Could you check a few things on this model? Use its own coordinates, in mm. A direction names the side the tool comes from. Coordinates: 2 decimals unless noted, no trailing zeros. Order: outer loops, then holes, each group sorted by start corner. A loop starts at its lowest first (then second) coordinate and runs counter-clockwise, first axis right, second up. Notation, with made-up numbers: (50, 72.25) -> (99, 72.25) arc R19 cw to (99, 100.25) -> close; hole circle Ø5 at (13, 18). An arc over 180 degrees is marked (long way). Use a Markdown table: item, result. Add a question column.
1) If we section it at B-B (y = 3): Write out the boundary of the cut face in (x, z), plus the area to 3 significant figures.
2) If we section it at A-A (z = 1.8): Write out the boundary of the cut face in (x, y).
3) Will these pins go through, and if not, where does the flat tip stop? pin 1 Ø8 at (x, y) = (-7, 5.5) entering from +Z; pin 2 Ø3 at (x, y) = (4.5, -5) entering from -Z.
4) If we section it at C-C (x = 2.25): Write out the boundary of the cut face in (y, z).
5) If I drill on L1, parallel to Z at x = -0.5, y = 1.25; L2, parallel to X at y = 6.75, z = 0.6; L3, parallel to Y at x = 5.5, z = 2.4, over which ranges is the centre line in solid material (lowest first)? Write a range as [from, to].
6) Which directions (+Z, -Z, +X, -X, +Y, -Y) give clear straight access to the entire face, cutting with the end or side of a thin tool? Please do faces 1 (the flat face through (9.1, 0, 2)), 2 (the cylindrical face through (0.323, 0.506, 3.569)).
```python
from build123d import *

# Parameters (mm, degrees)
BOSS_EXTRU_1_DEPTH = 3.15
ESQUISSE4_R        = 0.6
BOSS_EXTRU_2_DEPTH = 0.85
ESQUISSE5_R        = 0.35
BOSS_EXTRU_3_DEPTH = 0.4
ESQUISSE6_R        = 0.085
BOSS_EXTRU_4_DEPTH = 0.35


with BuildPart() as part:
    # Esquisse2 → Boss.-Extru.1 (new body)
    with BuildSketch(Plane.XY):
        with BuildLine():
            Line((9.1, 1.659066002), (9.1, -1.659066002))
            ThreePointArc((9.1, -1.659066002), (8.871356868, -2.619451721), (8.541662602, -3.55))
            Line((8.541662602, -3.55), (3.348120127, -6.7))
            Line((3.348120127, -6.7), (-3.348120127, -6.7))
            Line((-3.348120127, -6.7), (-8.541662602, -3.55))
            ThreePointArc((-8.541662602, -3.55), (-8.871356868, -2.619451721), (-9.1, -1.659066002))
            Line((-9.1, -1.659066002), (-9.1, 1.659066002))
            ThreePointArc((-9.1, 1.659066002), (-8.871356868, 2.619451721), (-8.541662602, 3.55))
            Line((-8.541662602, 3.55), (-2.441311123, 7.25))
            ThreePointArc((-2.441311123, 7.25), (0, 7.65), (2.441311123, 7.25))
            Line((2.441311123, 7.25), (8.541662602, 3.55))
            ThreePointArc((8.541662602, 3.55), (8.871356868, 2.619451721), (9.1, 1.659066002))
        make_face()
    extrude(amount=BOSS_EXTRU_1_DEPTH)

    # Esquisse4 → Boss.-Extru.2 (add)
    with BuildSketch(Plane.XY.offset(3.15)):
        Circle(ESQUISSE4_R)
    extrude(amount=BOSS_EXTRU_2_DEPTH)

    # Esquisse5 → Boss.-Extru.3 (add)
    with BuildSketch(Plane.XY.offset(4)):
        Circle(ESQUISSE5_R)
    extrude(amount=BOSS_EXTRU_3_DEPTH)

    # Esquisse6 → Boss.-Extru.4 (add)
    with BuildSketch(Plane.XY.offset(4.4)):
        Circle(ESQUISSE6_R)
    extrude(amount=BOSS_EXTRU_4_DEPTH)


solid = part.part
```
Answer sheet:
| question | item | result |
|---|---|---|
| 1 | outline | (-8.75, 0) -> (8.75, 0) -> (8.75, 3.15) -> (-8.75, 3.15) -> close |
| 1 | area | 55.1 mm2 |
| 2 | outline | (-9.1, -1.66) arc R9.25 ccw to (-8.54, -3.55) -> (-3.35, -6.7) -> (3.35, -6.7) -> (8.54, -3.55) arc R9.25 ccw to (9.1, -1.66) -> (9.1, 1.66) arc R9.25 ccw to (8.54, 3.55) -> (2.44, 7.25) arc R7.65 ccw to (-2.44, 7.25) -> (-8.54, 3.55) arc R9.25 ccw to (-9.1, 1.66) -> close |
| 3 | pin 1 | z = 3.15 |
| 3 | pin 2 | z = 0 |
| 4 | outline | (-6.7, 0) -> (7.31, 0) -> (7.31, 3.15) -> (-6.7, 3.15) -> close |
| 5 | L1 | [0, 3.15] |
| 5 | L2 | [-3.27, 3.27] |
| 5 | L3 | [-5.39, 5.39] |
| 6 | face 1 | +Z, -Z, +X, +Y, -Y |
| 6 | face 2 | +Z |
